Here's how the part is built. I have some questions about the finished solid (model axes, mm). Round coordinates to 2 decimals unless told otherwise and drop trailing zeros. Order: outer loops, then holes, each group sorted by start corner. A loop starts at its lowest first (then second) coordinate and runs counter-clockwise, first axis right, second up.
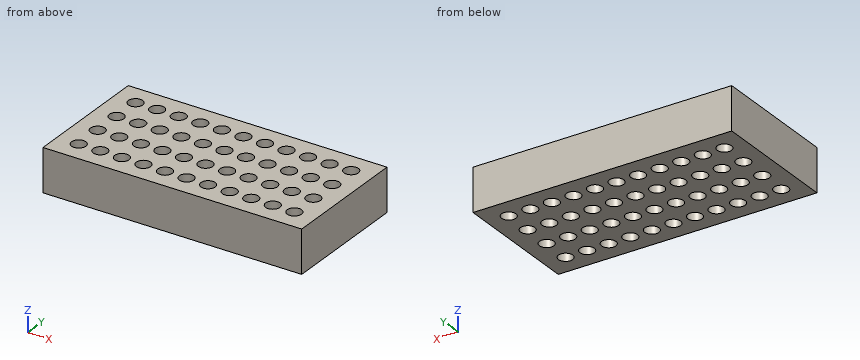
```python
from build123d import *

# Parameters (mm, degrees)
ESBO_O1_W                = 180
ESBO_O1_H                = 90
RESSALTO_EXTRUS_O1_DEPTH = 30
ESBO_O2_R                = 5
CORTE_EXTRUS_O1_DEPTH    = 30


with BuildPart() as part:
    # Esboço1 → Ressalto-extrusão1 (new body)
    with BuildSketch(Plane.XY):
        Rectangle(ESBO_O1_W, ESBO_O1_H)
    extrude(amount=RESSALTO_EXTRUS_O1_DEPTH)

    # Esboço2 → Corte-extrusão1 (cut)
    with BuildSketch(Plane.XY.offset(30)):
        with Locations((-75, 30)):
            Circle(ESBO_O2_R)
        with Locations((-60, 30)):
            Circle(ESBO_O2_R)
        with Locations((-45, 30)):
            Circle(ESBO_O2_R)
        with Locations((-30, 30)):
            Circle(ESBO_O2_R)
        with Locations((-15, 30)):
            Circle(ESBO_O2_R)
        with Locations((0, 30)):
            Circle(ESBO_O2_R)
        with Locations((15, 30)):
            Circle(ESBO_O2_R)
        with Locations((30, 30)):
            Circle(ESBO_O2_R)
        with Locations((45, 30)):
            Circle(ESBO_O2_R)
        with Locations((60, 30)):
            Circle(ESBO_O2_R)
        with Locations((75, 30)):
            Circle(ESBO_O2_R)
        with Locations((-60, 10)):
            Circle(ESBO_O2_R)
        with Locations((-45, 10)):
            Circle(ESBO_O2_R)
        with Locations((-30, 10)):
            Circle(ESBO_O2_R)
        with Locations((-15, 10)):
            Circle(ESBO_O2_R)
        with Locations((0, 10)):
            Circle(ESBO_O2_R)
        with Locations((15, 10)):
            Circle(ESBO_O2_R)
        with Locations((30, 10)):
            Circle(ESBO_O2_R)
        with Locations((45, 10)):
            Circle(ESBO_O2_R)
        with Locations((60, 10)):
            Circle(ESBO_O2_R)
        with Locations((75, 10)):
            Circle(ESBO_O2_R)
        with Locations((-60, -10)):
            Circle(ESBO_O2_R)
        with Locations((-45, -10)):
            Circle(ESBO_O2_R)
        with Locations((-30, -10)):
            Circle(ESBO_O2_R)
        with Locations((-15, -10)):
            Circle(ESBO_O2_R)
        with Locations((0, -10)):
            Circle(ESBO_O2_R)
        with Locations((15, -10)):
            Circle(ESBO_O2_R)
        with Locations((30, -10)):
            Circle(ESBO_O2_R)
        with Locations((45, -10)):
            Circle(ESBO_O2_R)
        with Locations((60, -10)):
            Circle(ESBO_O2_R)
        with Locations((75, -10)):
            Circle(ESBO_O2_R)
        with Locations((-60, -30)):
            Circle(ESBO_O2_R)
        with Locations((-45, -30)):
            Circle(ESBO_O2_R)
        with Locations((-30, -30)):
            Circle(ESBO_O2_R)
        with Locations((-15, -30)):
            Circle(ESBO_O2_R)
        with Locations((0, -30)):
            Circle(ESBO_O2_R)
        with Locations((15, -30)):
            Circle(ESBO_O2_R)
        with Locations((30, -30)):
            Circle(ESBO_O2_R)
        with Locations((45, -30)):
            Circle(ESBO_O2_R)
        with Locations((60, -30)):
            Circle(ESBO_O2_R)
        with Locations((75, -30)):
            Circle(ESBO_O2_R)
        with Locations((-75, 10)):
            Circle(ESBO_O2_R)
        with Locations((-75, -10)):
            Circle(ESBO_O2_R)
        with Locations((-75, -30)):
            Circle(ESBO_O2_R)
    extrude(amount=-CORTE_EXTRUS_O1_DEPTH, mode=Mode.SUBTRACT)


solid = part.part
```
1. I need wall thicknesses on probe 1 along Y at (x, z) = (-75, 10.5); probe 2 along Y at (x, z) = (-2.5, 19.5). Which ranges of each line are inside material? Lowest first, please.
Evaluation:
probe 1: y = -45 to -35, -25 to -15, -5 to 5, 15 to 25, 35 to 45
probe 2: y = -45 to -34.33, -25.67 to -14.33, -5.67 to 5.67, 14.33 to 25.67, 34.33 to 45
2. If we section it at A-A, the plane x = -33: Write out the boundary of the cut face in (y, z).
Evaluation:
outline: (-45, 0) - (-34, 0) - (-34, 30) - (-45, 30) - close; (-26, 0) - (-14, 0) - (-14, 30) - (-26, 30) - close; (-6, 0) - (6, 0) - (6, 30) - (-6, 30) - close; (14, 0) - (26, 0) - (26, 30) - (14, 30) - close; (34, 0) - (45, 0) - (45, 30) - (34, 30) - close
3. If we section it at B-B, the plane y = 13: State how many separate pieces and enclosed holes the cut face has, and give its area (3 significant figures).
Evaluation:
separate pieces: 12
enclosed holes: 0
area: 2,760 mm2
4. If we section it at D-D, the plane x = -60: Write out the boundary of the cut face in (y, z).
Evaluation:
outline: (-45, 0) - (-35, 0) - (-35, 30) - (-45, 30) - close; (-25, 0) - (-15, 0) - (-15, 30) - (-25, 30) - close; (-5, 0) - (5, 0) - (5, 30) - (-5, 30) - close; (15, 0) - (25, 0) - (25, 30) - (15, 30) - close; (35, 0) - (45, 0) - (45, 30) - (35, 30) - close
